Input: part model. Units: mm. Frame: model coordinates. Face numbers are marked on the shaded views. A direction names the side the tool comes from. Coordinates: 2 decimals unless noted, no trailing zeros. Order: outer loops, then holes, each group sorted by start corner. A loop starts at its lowest first (then second) coordinate and runs counter-clockwise, first axis right, second up. Notation, with made-up numbers: (64, 29) - (106, 29) arc R13 cw to (106, 39) - close; hole circle Ø5 at (53, 7). An arc over 180 degrees is marked (long way). Use a Markdown table: item, result. Add a question column.
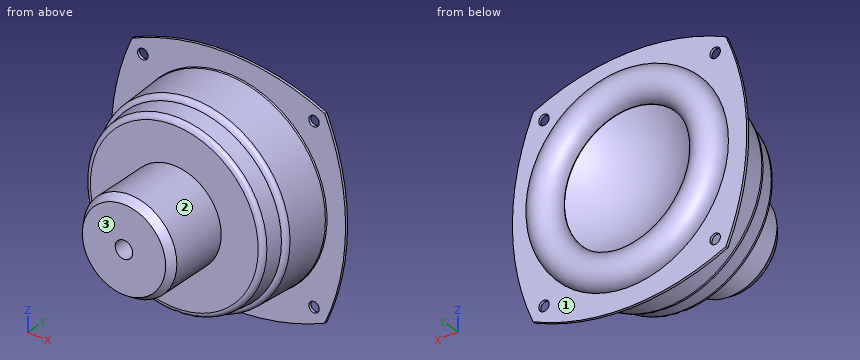
from build123d import *

# Parameters (mm, degrees)
F1_DEPTH  = 1
F2_R      = 37.75
F3_DEPTH  = 19
F4_SIZE2  = 18.99999
F4_SIZE   = 0.99999
F5_R      = 35
F6_DEPTH  = 8
F7_SIZE2  = 7.99999
F7_SIZE   = 0.99999
F9_R      = 2
F10_R     = 18
F11_DEPTH = 25.1
F12_SIZE2 = 3
F12_SIZE  = 2
F13_R     = 3.3621070756
F14_DEPTH = 25
F15_R     = 2
F16_DEPTH = 53.101
F19_R     = 6.5


# Not quite as in the source:
# - a fillet or chamfer that OpenCascade refuses, or shapes differently, is made with other operations: its cross-section is extruded or revolved along the edge and cut away or added
# - a fillet or chamfer is up to 0.001 mm smaller than in the source, because OpenCascade refuses the exact size


with BuildPart() as f1:
    # F0 (on Front) → F1 (new body)
    with BuildSketch(Plane.XZ):
        with BuildLine():
            ThreePointArc((37.029404499, -37.029404499), (45, 0), (37.029404499, 37.029404499))
            ThreePointArc((37.029404499, 37.029404499), (0, 45), (-37.029404499, 37.029404499))
            ThreePointArc((-37.029404499, 37.029404499), (-45, 0), (-37.029404499, -37.029404499))
            ThreePointArc((-37.029404499, -37.029404499), (0, -45), (37.029404499, -37.029404499))
        make_face()
    extrude(amount=F1_DEPTH)

    # F2 (on face) → F3 (join)
    with BuildSketch(Plane.XZ.offset(1)):
        Circle(F2_R)
    extrude(amount=F3_DEPTH)

    # F4 (size 1 and 19 in the source; OpenCascade refuses exactly that, so slightly less here)
    f4_edges = [f1.edges().sort_by_distance(p)[0] for p in [
        (-37.75, -20, 0),
    ]]
    f4_side = f1.faces().sort_by_distance((0, -20, 0))[0]
    chamfer(f4_edges, length=F4_SIZE, length2=F4_SIZE2, reference=f4_side)

    # F5 (on face) → F6 (join)
    with BuildSketch(Plane.XZ.offset(20)):
        Circle(F5_R)
    extrude(amount=F6_DEPTH)

    # F7 (size 1 and 8 in the source; OpenCascade refuses exactly that, so slightly less here)
    f7_edges = [f1.edges().sort_by_distance(p)[0] for p in [
        (-35, -28, 0),
    ]]
    f7_side = f1.faces().sort_by_distance((0, -28, 0))[0]
    chamfer(f7_edges, length=F7_SIZE, length2=F7_SIZE2, reference=f7_side)

    # F8: fillet of radius 2 on 1 edges, made by hand

    # F8_s1 → F8_t2 (revolve, cut)
    with BuildSketch(Plane.XY):
        with BuildLine():
            ThreePointArc((35, -20), (36.2814643906, -19.4044849409), (36.8494519972, -18.110584153))
            Line((36.8494519972, -18.110584153), (36.8893967114, -18.1126864865))
            Line((36.8893967114, -18.1126864865), (36.7899547142, -20.0021023335))
            Line((36.7899547142, -20.0021023335), (36.75001, -20.04))
            ThreePointArc((36.75001, -20.04), (35.875005, -20.04), (35.0029556743, -20.0398906504))
            Line((35.0029556743, -20.0398906504), (35, -20))
        make_face()
    revolve(axis=Axis((0, -20, 0), (0, -1, 0)), mode=Mode.SUBTRACT)

    # F9
    f9_edges = [f1.edges().sort_by_distance(p)[0] for p in [
        (-34.00001, -28, 0),
    ]]
    fillet(f9_edges, radius=F9_R)

    # F10 (on face) → F11 (join)
    with BuildSketch(Plane.XZ.offset(28)):
        Circle(F10_R)
    extrude(amount=F11_DEPTH)

    # F12
    f12_edges = [f1.edges().sort_by_distance(p)[0] for p in [
        (-18, -53.1, 0),
    ]]
    f12_side = f1.faces().sort_by_distance((0, -53.1, 0))[0]
    chamfer(f12_edges, length=F12_SIZE, length2=F12_SIZE2, reference=f12_side)

    # F13 (on face) → F14 (cut)
    with BuildSketch(Plane.XZ.offset(53.1)):
        Circle(F13_R)
    extrude(amount=-F14_DEPTH, mode=Mode.SUBTRACT)

    # F15 (on face) → F16 (cut, through all)
    with BuildSketch(Plane(origin=(0, 0, 0), x_dir=(-1, 0, 0), z_dir=(0, 1, 0))):
        with Locations((-32.8804653252, 32.8804653252)):
            Circle(F15_R)
        with Locations((-32.8804653252, -32.8804653252)):
            Circle(F15_R)
        with Locations((32.8804653252, -32.8804653252)):
            Circle(F15_R)
        with Locations((32.8804653252, 32.8804653252)):
            Circle(F15_R)
    extrude(amount=-F16_DEPTH, mode=Mode.SUBTRACT)

    # F17 (on Top) → F18 (revolve, cut)
    with BuildSketch(Plane.XY):
        with BuildLine():
            Line((0, 0), (-25, 0))
            ThreePointArc((-25, 0), (-13.3392655896, -6.9096080905), (0, -9.3136472921))
            Line((0, -9.3136472921), (0, 0))
        make_face()
    revolve(axis=Axis((0, 14.4480448216, 0), (0, 1, 0)), mode=Mode.SUBTRACT)

    # F19 (on Top) → F20 (revolve)
    with BuildSketch(Plane.XY):
        with Locations((-31.4735865454, 0.2)):
            Circle(F19_R)
    revolve(axis=Axis((0, 14.4480448216, 0), (0, 1, 0)))


solid = f1.part
1) Material intervals for L1, parallel to Z at x = 0, y = -36; L2, parallel to Y at x = -29.5, z = -29; L3, parallel to X at y = 1.5, z = -21, sorted ascending.
2) Contact query for flat-ended pins moving along their axis: P1, Ø1.5, axis at y = -2.5, z = 14, coming from the +X side; P2, Ø12, axis at y = -32.5, z = -16, coming from the -X side; P3, Ø5.5, axis at x = 0, z = 0, coming from the -Y side. Output: stop coordinate, or through.
3) Reachability of the marked faces 1, 2 and 3 from +Z, -Z, +X, -X, +Y, -Y: full face, straight path, thin tool, end or side. Return the list, or none.
4) Cut plane B-B (y = -7.5). Return the cut outline in (x, z).
Computed:
| question | item | result |
|---|---|---|
| 1 | L1 | z = -18 to -3.36, 3.36 to 18 |
| 1 | L2 | y = -1 to 0 |
| 1 | L3 | x = -31.48 to -13.76, 13.76 to 31.48 |
| 2 | P1 | stops at x = 35.27 |
| 2 | P2 | stops at x = -31.16 |
| 2 | P3 | stops at y = -28.1 |
| 3 | face 1 | +Y |
| 3 | face 2 | -Y |
| 3 | face 3 | +Z, -Z, +X, -X, -Y |
| 4 | outline | circle Ø74.82 at (0, 0); hole circle Ø23.26 at (0, 0) |
